Geometry check sheet. Reference: drawing and pictorial views, mm from the part's lowest x, y, z. Round coordinates to 2 decimals unless told otherwise and drop trailing zeros. Order: outer loops, then holes, each group sorted by start corner. A loop starts at its lowest first (then second) coordinate and runs counter-clockwise, first axis right, second up.
(1) Cross-section at A-A on y = 6. Enter the section's corners in (x, z), and give its area (4 significant figures).
(2) Gauge pin test, flat ends, axial feed: P1, Ø1, axis at y = 5.5, z = 13.5, coming from the +X side; P2, Ø2, axis at y = 5, z = 33, coming from the +X side; P3, Ø4.5, axis at y = 6.5, z = 35, coming from the -X side. Record the tip position at first contact, or that the pin passes through.
(3) Draft check along Y on the marked faces 1 and 2. Enter one of: pulls with the +Y half, pulls with the -Y half, needs draft (parallel to the pull), parting line crosses it, or undercut.
(4) Thickness scan on L1, parallel to Z at x = 79, y = 7.5; L2, parallel to Y at x = 27.5, z = 9.5; L3, parallel to X at y = 5.75, z = 3. Record the ranges inside material, lowest first.
(5) Cross-section at C-C on z = 37.5. Enter the section's corners in (x, y).
(6) Cross-section at B-B on x = 86. Enter the section's corners in (y, z).
(7) Cross-section at D-D on z = 47.5. Enter the section's corners in (x, y), and give its area (3 significant figures).
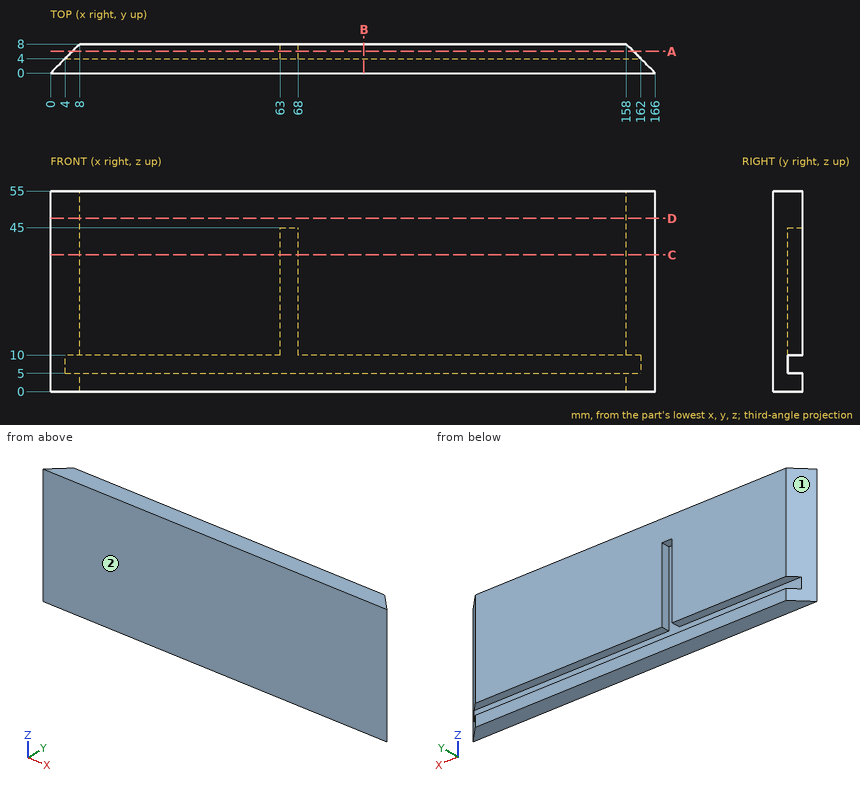
Found:
1. outline: (6, 0) - (160, 0) - (160, 5) - (6, 5) - close; (6, 10) - (63, 10) - (63, 45) - (68, 45) - (68, 10) - (160, 10) - (160, 55) - (6, 55) - close
1. area: 7,525 mm2
2. P1: stops at x = 161
2. P2: stops at x = 162
2. P3: stops at x = 4.25
3. face 1: pulls with the +Y half
3. face 2: pulls with the -Y half
4. L1: z = 0 to 5, 10 to 55
4. L2: y = 0 to 4
4. L3: x = 5.75 to 160.25
5. outline: (0, 0) - (166, 0) - (158, 8) - (68, 8) - (68, 4) - (63, 4) - (63, 8) - (8, 8) - close
6. outline: (0, 0) - (8, 0) - (8, 5) - (4, 5) - (4, 10) - (8, 10) - (8, 55) - (0, 55) - close
7. outline: (0, 0) - (166, 0) - (158, 8) - (8, 8) - close
7. area: 1,260 mm2
